Here's how the part is built. I have some questions about the finished solid (model axes, mm). A direction names the side the tool comes from. Give positions to 0.01 mm unless a question says otherwise; leave off trailing zeros. Write each loop counter-clockwise with the first axis right and the second up, starting at its lowest first coordinate (ties: lowest second). Pieces come first, ordered by that corner, then holes. Notation, with made-up numbers: (70.5, -27) -> (96.5, -27) arc R19 ccw to (96.5, -21) -> close; hole circle Ø10 at (-21, 9.5). An arc over 180 degrees is marked (long way). Use CSV: the item, a comma, the result in double quotes. Start each with the question number.
(1) Suppose I cut it at C-C on y = 8.25. List the corners of the cut face in (x, z) for me, plus the area to 3 significant figures.
(2) Suppose I cut it at B-B on z = 0. List the corners of the cut face in (x, y) for me, plus the area to 3 significant figures.
(3) Suppose I cut it at A-A on x = 0. List the corners of the cut face in (y, z) for me, plus the area to 3 significant figures.
(4) For pin 1 Ø1 at (x, y) = (-2.5, 8.5) entering from +Z; pin 2 Ø1.5 at (x, z) = (-2.5, 1.5) entering from -Y; pin 3 Ø4 at (y, z) = (7.5, -3.5) entering from -X, each with a flat end and sliding along its axis, tell me the tip position at first contact or that it passes through.
(5) Suppose I cut it at D-D on y = 1.75. List the corners of the cut face in (x, z) for me.
(6) If we mould it in two halves opening along Z, with no side actions, what happens to faces 3 (the flat face through (0, 12, 6)), 4 (the cylindrical face through (0.66, 6.119, -14.985)), 5 (the flat face through (-2, 7.5, -4)), 6 (the cylindrical face through (-3.905, 3.698, -0.867))? For each: pulls with the +Z half, pulls with the -Z half, needs draft (parallel to the pull), parting line crosses it, or undercut.
(7) Which directions (+Z, -Z, +X, -X, +Y, -Y) give clear straight access to the entire face, cutting with the end or side of a thin tool? Please do faces 1 (the flat face through (-3, 0, 3)), 2 (the cylindrical face through (-5.37, 9.78, -1.19)).
(8) I need wall thicknesses on L1, parallel to X at y = 10.45, z = 0; L2, parallel to X at y = 4, z = 0; L3, parallel to Z at x = 3.5, y = 3. Which ranges of each line are inside material? Lowest first, please. Write a range as [from, to].
from build123d import *

# Parameters (mm, degrees)
SKETCH1_R           = 15
SKETCH1_R_2         = 4
BOSS_EXTRUDE1_DEPTH = 12
SKETCH2_R           = 5.5
CUT_EXTRUDE1_DEPTH  = 4.5
CHAMFER1_SIZE       = 0.4
CHAMFER1_SIZE2      = 0.399999869


with BuildPart() as part:
    # Sketch1 → Boss-Extrude1 (new body)
    with BuildSketch(Plane(origin=(0, 0, 0), x_dir=(1, 0, 0), z_dir=(0, 1, 0))):
        with Locations(Location((0, 0, 0), (0, 0, 270))):
            Circle(SKETCH1_R)
        with Locations(Location((0, 0, 0), (0, 0, 270))):
            Circle(SKETCH1_R_2, mode=Mode.SUBTRACT)
    extrude(amount=BOSS_EXTRUDE1_DEPTH)

    # Sketch2 → Cut-Extrude1 (cut, symmetric)
    with BuildSketch(Plane(origin=(0, 12, 0), x_dir=(1, 0, 0), z_dir=(0, 1, 0))):
        with Locations(Location((0, 0, 0), (0, 0, 270))):
            Circle(SKETCH2_R)
    extrude(amount=CUT_EXTRUDE1_DEPTH, both=True, mode=Mode.SUBTRACT)

    # Chamfer1
    chamfer1_edges = [part.edges().sort_by_distance(p)[0] for p in [
        (0, 0, -15),
    ]]
    chamfer1_side = [part.faces().sort_by_distance(p)[0] for p in [
        (0, 6, -15),
    ]]
    chamfer(chamfer1_edges, length=CHAMFER1_SIZE, length2=CHAMFER1_SIZE2, reference=chamfer1_side[0])


solid = part.part
Geometry says:
1,outline,"circle Ø30 at (0, 0); hole circle Ø11 at (0, 0)"
1,area,"612 mm²"
2,outline,"(-15, 0.4) -> (-14.6, 0) -> (-4, 0) -> (-4, 7.5) -> (-5.5, 7.5) -> (-5.5, 12) -> (-15, 12) -> close; (4, 0) -> (14.6, 0) -> (15, 0.4) -> (15, 12) -> (5.5, 12) -> (5.5, 7.5) -> (4, 7.5) -> close"
2,area,"250 mm²"
3,outline,"(0, -14.6) -> (0.4, -15) -> (12, -15) -> (12, -5.5) -> (7.5, -5.5) -> (7.5, -4) -> (0, -4) -> close; (0, 4) -> (7.5, 4) -> (7.5, 5.5) -> (12, 5.5) -> (12, 15) -> (0.4, 15) -> (0, 14.6) -> close"
3,area,"250 mm²"
4,pin 1,"z = 14.87"
4,pin 2,"through"
4,pin 3,"x = -14.92"
5,outline,"circle Ø30 at (0, 0); hole circle Ø8 at (0, 0)"
6,face 3,"needs draft"
6,face 4,"parting line crosses it"
6,face 5,"undercut"
6,face 6,"undercut"
7,face 1,"+Z, -Z, +X, -X, -Y"
7,face 2,"+Y"
8,L1,"[-15, -5.5], [5.5, 15]"
8,L2,"[-15, -4], [4, 15]"
8,L3,"[-14.59, -1.94], [1.94, 14.59]"
